Part model, mm, in its own coordinate system. Face numbers are marked on the shaded views. A direction names the side the tool comes from. Round coordinates to 2 decimals unless told otherwise and drop trailing zeros. Write each loop counter-clockwise with the first axis right and the second up, starting at its lowest first coordinate (ties: lowest second). Pieces come first, ordered by that corner, then holes. Notation, with made-up numbers: M 63,29 L 122,29 A21 ccw 122,60 Z; hole C 5,73 d1. An arc over 180 degrees is marked long. One line per question, with ' | ' between items. Start each with the question number.
1) Saw through at A-A (y = 5.5). List the corners of the cut face in (x, z).
2) Mould opens along X. For the marked faces 1, 2 and 3 say: pulls with the +X half, pulls with the -X half, needs draft (parallel to the pull), parting line crosses it, or undercut.
3) Saw through at B-B (z = 14). List the corners of the cut face in (x, y), plus the area to 3 significant figures.
4) Saw through at D-D (z = 7.5). List the corners of the cut face in (x, y).
5) Tool access for the marked faces 4, 5, 6, 7 and 8: list every direction of +Z, -Z, +X, -X, +Y, -Y with a clear straight run to the whole face (end or side of a thin tool).
6) Saw through at C-C (x = 0). List the corners of the cut face in (y, z).
7) Wall check: probe 1 along Y at (x, z) = (-17, 24); probe 2 along X at (y, z) = (24, 30); probe 3 along X at (y, z) = (3, 20). Give the ranges that are in metal, low to high. Write a range as [from, to].
8) Drop flat-ended pins along their axis: pin 1 Ø7.5 at (x, y) = (10, 10) entering from +Z; pin 2 Ø5 at (x, y) = (13, 15.5) entering from -Z; pin 3 Ø14 at (x, z) = (5.5, 17.5) entering from +Y. Give the stop position or say it passes through.
```python
from build123d import *

# Parameters (mm, degrees)
PAD_DEPTH    = 28
SKETCH001_W  = 30
SKETCH001_H  = 36
PAD001_DEPTH = 3
SKETCH002_R  = 2.5
PAD002_DEPTH = 4


with BuildPart() as part:
    # Sketch → Pad (new body)
    with BuildSketch(Plane.XY):
        with BuildLine():
            Line((-20, 15), (20, 15))
            Line((20, 15), (20, 0))
            Line((20, 0), (11, -2.2e-05))
            ThreePointArc((11, -2.2e-05), (1.1e-05, 11), (-11, 0))
            Line((-11, 0), (-20, 0))
            Line((-20, 0), (-20, 15))
        make_face()
    extrude(amount=PAD_DEPTH)

    # Sketch001 (on Face6 of Pad) → Pad001 (join)
    with BuildSketch(Plane(origin=(-20, 0, 0), x_dir=(0, -1, 0), z_dir=(-1, 0, 0))):
        with Locations((-15, 14)):
            Rectangle(SKETCH001_W, SKETCH001_H)
    extrude(amount=PAD001_DEPTH)

    # Sketch002 (on Face5 of Pad001) → Pad002 (join)
    with BuildSketch(Plane(origin=(-23, 0, 0), x_dir=(0, -1, 0), z_dir=(-1, 0, 0))):
        with Locations((-12.5, 14)):
            Circle(SKETCH002_R)
    extrude(amount=PAD002_DEPTH)


solid = part.part
```
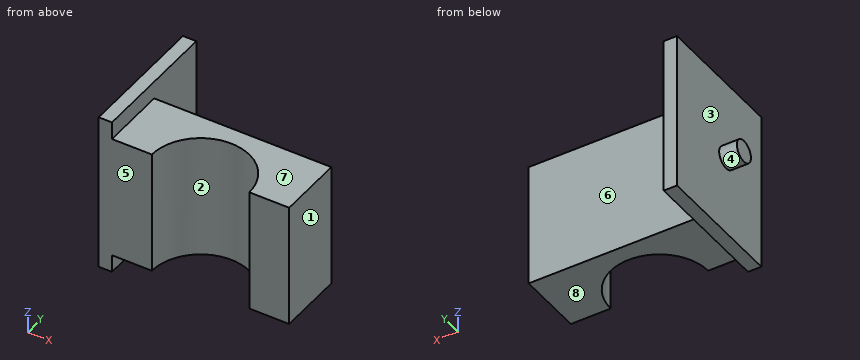
Answer key:
1) outline: M -23,-4 L -20,-4 L -20,0 L -9.53,0 L -9.53,28 L -20,28 L -20,32 L -23,32 Z; M 9.53,0 L 20,0 L 20,28 L 9.53,28 Z
2) face 1: pulls with the +X half | face 2: undercut | face 3: pulls with the -X half
3) outline: M -27,10 L -23,10 L -23,0 L -11,0 A11 cw 11,0 L 20,0 L 20,15 L -20,15 L -20,30 L -23,30 L -23,15 L -27,15 Z | area: 520 mm2
4) outline: M -23,0 L -11,0 A11 cw 11,0 L 20,0 L 20,15 L -20,15 L -20,30 L -23,30 Z
5) face 4: -X | face 5: +Z, -Z, +X, -X, -Y | face 6: +Z, -Z, +X, +Y | face 7: +Z, +X, +Y, -Y | face 8: -Z, +X, +Y, -Y
6) outline: M 11,0 L 15,0 L 15,28 L 11,28 Z
7) probe 1: y = [0, 15] | probe 2: x = [-23, -20] | probe 3: x = [-23, -10.58], [10.58, 20]
8) pin 1: stops at z = 28 | pin 2: stops at z = 0 | pin 3: stops at y = 15
